Check sheet for the modelled part. Datum: model origin and axes. Units: mm. A direction names the side the tool comes from. Coordinates: 2 decimals unless noted, no trailing zeros. Loops run counter-clockwise (first coordinate to the right, second up) from the corner with the lowest first, then second, coordinate; pieces in that order, holes last.
```python
from build123d import *

# Parameters (mm, degrees)
SKETCH1_R              = 14.2875
SKETCH1_R_2            = 30
SKETCH1_R_3            = 15
SKETCH1_R_4            = 1.85
BOSS_EXTRUDE1_DEPTH    = 4
M3_5_CLEARANCE_HOLE1_D = 3.9
CUT_EXTRUDE1_DEPTH     = 10


with BuildPart() as part:
    # Sketch1 → Boss-Extrude1 (new body)
    with BuildSketch(Plane.XY):
        with BuildLine():
            Line((-228.151452703, 51.156245998), (232.657949662, 23.244899096))
            ThreePointArc((232.657949662, 23.244899096), (254.5375, 0), (232.657949662, -23.244899096))
            Line((232.657949662, -23.244899096), (-228.151452703, -51.156245998))
            ThreePointArc((-228.151452703, -51.156245998), (-282.5, 0), (-228.151452703, 51.156245998))
        make_face()
        with Locations((231.25, 0)):
            Circle(SKETCH1_R, mode=Mode.SUBTRACT)
        with Locations((-231.25, 0)):
            Circle(SKETCH1_R_2, mode=Mode.SUBTRACT)
        with Locations((-110.25, 0)):
            Circle(SKETCH1_R_3, mode=Mode.SUBTRACT)
        with Locations((-201.25, 44.517654426)):
            Circle(SKETCH1_R_4, mode=Mode.SUBTRACT)
        with Locations((-102.663346073, 38.546234825)):
            Circle(SKETCH1_R_4, mode=Mode.SUBTRACT)
        with Locations((-4.076692145, 32.574815224)):
            Circle(SKETCH1_R_4, mode=Mode.SUBTRACT)
        with Locations((94.509961782, 26.603395622)):
            Circle(SKETCH1_R_4, mode=Mode.SUBTRACT)
        with Locations((193.096615709, 20.631976021)):
            Circle(SKETCH1_R_4, mode=Mode.SUBTRACT)
        with Locations(Location((193.096615709, -20.631976021, 0), (0, 0, 180))):
            Circle(SKETCH1_R_4, mode=Mode.SUBTRACT)
        with Locations(Location((94.509961782, -26.603395622, 0), (0, 0, 180))):
            Circle(SKETCH1_R_4, mode=Mode.SUBTRACT)
        with Locations(Location((-4.076692145, -32.574815224, 0), (0, 0, 180))):
            Circle(SKETCH1_R_4, mode=Mode.SUBTRACT)
        with Locations(Location((-102.663346073, -38.546234825, 0), (0, 0, 180))):
            Circle(SKETCH1_R_4, mode=Mode.SUBTRACT)
        with Locations(Location((-201.25, -44.517654426, 0), (0, 0, 180))):
            Circle(SKETCH1_R_4, mode=Mode.SUBTRACT)
    extrude(amount=BOSS_EXTRUDE1_DEPTH)

    # M3.5 Clearance Hole1 (through all)
    with Locations(Plane.XY.offset(4)):
        with Locations((-231.25, 42.5), (-188.75, 0), (-132.75, 0), (-110.25, 22.5), (-87.75, 0), (-110.25, -22.5), (-273.75, 0), (-231.25, -42.5)):
            Hole(M3_5_CLEARANCE_HOLE1_D / 2)

    # Sketch7 → Cut-Extrude1 (cut)
    with BuildSketch(Plane.XY.offset(4)):
        with BuildLine():
            Line((108.094193191, 19.830412487), (152.959047941, 7.723728338))
            ThreePointArc((152.959047941, 7.723728338), (158.874816531, 0), (152.959047941, -7.723728338))
            Line((152.959047941, -7.723728338), (108.094193191, -19.830412487))
            ThreePointArc((108.094193191, -19.830412487), (101.145491167, -18.457819925), (98.009961782, -12.106684149))
            Line((98.009961782, -12.106684149), (98.009961782, 12.106684149))
            ThreePointArc((98.009961782, 12.106684149), (101.145491167, 18.457819925), (108.094193191, 19.830412487))
        make_face()
        with BuildLine():
            Line((91.009961782, -5.704410534), (91.009961782, 15.277961264))
            ThreePointArc((91.009961782, 15.277961264), (88.835311789, 20.761144399), (83.493637458, 23.263326493))
            Line((83.493637458, 23.263326493), (44.615483399, 25.618186527))
            ThreePointArc((44.615483399, 25.618186527), (36.490430728, 20.001229544), (40.014500476, 10.773682793))
            Line((40.014500476, 10.773682793), (78.892654535, -12.563549039))
            ThreePointArc((78.892654535, -12.563549039), (86.950871704, -12.666395092), (91.009961782, -5.704410534))
        make_face()
        with BuildLine():
            Line((11.040615102, 18.835101612), (59.256061992, -10.106989112))
            ThreePointArc((59.256061992, -10.106989112), (62.909345697, -18.868209702), (55.62243042, -24.951492846))
            Line((55.62243042, -24.951492846), (7.40698353, -27.871915166))
            ThreePointArc((7.40698353, -27.871915166), (1.440124719, -25.711899944), (-1.076692145, -19.886549937))
            Line((-1.076692145, -19.886549937), (-1.076692145, 11.975963107))
            ThreePointArc((-1.076692145, 11.975963107), (2.982397933, 18.937947665), (11.040615102, 18.835101612))
        make_face()
        with BuildLine():
            Line((-7.076692145, -16.488216766), (-7.076692145, 16.488216766))
            ThreePointArc((-7.076692145, 16.488216766), (-10.56107203, 23.091941092), (-17.978985888, 23.943194367))
            Line((-17.978985888, 23.943194367), (-60.331448304, 7.454977601))
            ThreePointArc((-60.331448304, 7.454977601), (-65.429154561, 0), (-60.331448304, -7.454977601))
            Line((-60.331448304, -7.454977601), (-17.978985888, -23.943194367))
            ThreePointArc((-17.978985888, -23.943194367), (-10.56107203, -23.091941092), (-7.076692145, -16.488216766))
        make_face()
        with BuildLine():
            Line((-79.023457852, 6.616651493), (-41.387349534, 21.268746715))
            ThreePointArc((-41.387349534, 21.268746715), (-38.261519247, 26.701886011), (-42.898985826, 30.918960984))
            Line((-42.898985826, 30.918960984), (-98.34861526, 34.277559647))
            ThreePointArc((-98.34861526, 34.277559647), (-103.531708107, 30.371987358), (-100.492037548, 24.638022826))
            ThreePointArc((-100.492037548, 24.638022826), (-91.408821848, 18.634913625), (-85.506059466, 9.486169241))
            ThreePointArc((-85.506059466, 9.486169241), (-82.861226958, 6.703913435), (-79.023457852, 6.616651493))
        make_face()
        with BuildLine():
            Line((-172.485050673, 29.401404781), (-141.465979865, 9.242335075))
            ThreePointArc((-141.465979865, 9.242335075), (-137.374294793, 8.625273291), (-134.218916995, 11.302257212))
            ThreePointArc((-134.218916995, 11.302257212), (-127.488882583, 20.126373923), (-117.7355471, 25.420790401))
            ThreePointArc((-117.7355471, 25.420790401), (-114.065979457, 30.952175342), (-118.881140508, 35.52122011))
            Line((-118.881140508, 35.52122011), (-169.458127675, 38.584681548))
            ThreePointArc((-169.458127675, 38.584681548), (-174.509115504, 35.159056133), (-172.485050673, 29.401404781))
        make_face()
        with BuildLine():
            Line((-192.622687213, 24.889664687), (-187.500750367, 6.648335526))
            ThreePointArc((-187.500750367, 6.648335526), (-185.706988459, 4.01513348), (-182.686915809, 3))
            Line((-182.686915809, 3), (-159.740638738, 3))
            ThreePointArc((-159.740638738, 3), (-154.946782383, 6.579105474), (-157.016013037, 12.192423498))
            Line((-157.016013037, 12.192423498), (-185.084226954, 30.43375266))
            ThreePointArc((-185.084226954, 30.43375266), (-190.771187254, 30.269303059), (-192.622687213, 24.889664687))
        make_face()
        with BuildLine():
            Line((-118.881140508, -35.52122011), (-169.458127675, -38.584681548))
            ThreePointArc((-169.458127675, -38.584681548), (-174.509115504, -35.159056133), (-172.485050673, -29.401404781))
            Line((-172.485050673, -29.401404781), (-141.465979865, -9.242335075))
            ThreePointArc((-141.465979865, -9.242335075), (-137.374294793, -8.625273291), (-134.218916995, -11.302257212))
            ThreePointArc((-134.218916995, -11.302257212), (-127.488882583, -20.126373923), (-117.7355471, -25.420790401))
            ThreePointArc((-117.7355471, -25.420790401), (-114.065979457, -30.952175342), (-118.881140508, -35.52122011))
        make_face()
        with BuildLine():
            Line((-157.016013037, -12.192423498), (-185.084226954, -30.43375266))
            ThreePointArc((-185.084226954, -30.43375266), (-190.771187254, -30.269303059), (-192.622687213, -24.889664687))
            Line((-192.622687213, -24.889664687), (-187.500750367, -6.648335526))
            ThreePointArc((-187.500750367, -6.648335526), (-185.706988459, -4.01513348), (-182.686915809, -3))
            Line((-182.686915809, -3), (-159.740638738, -3))
            ThreePointArc((-159.740638738, -3), (-154.946782383, -6.579105474), (-157.016013037, -12.192423498))
        make_face()
        with BuildLine():
            Line((-42.898985826, -30.918960984), (-98.34861526, -34.277559647))
            ThreePointArc((-98.34861526, -34.277559647), (-103.531708107, -30.371987358), (-100.492037548, -24.638022826))
            ThreePointArc((-100.492037548, -24.638022826), (-91.408821848, -18.634913625), (-85.506059466, -9.486169241))
            ThreePointArc((-85.506059466, -9.486169241), (-82.861226958, -6.703913435), (-79.023457852, -6.616651493))
            Line((-79.023457852, -6.616651493), (-41.387349534, -21.268746715))
            ThreePointArc((-41.387349534, -21.268746715), (-38.261519247, -26.701886011), (-42.898985826, -30.918960984))
        make_face()
    extrude(amount=-CUT_EXTRUDE1_DEPTH, mode=Mode.SUBTRACT)


solid = part.part
```
1) Section check B-B on x = 27.5. Enter the section's corners in (y, z).
Answer sheet:
outline: (-35.67, 0) - (-26.65, 0) - (-26.65, 4) - (-35.67, 4) - close; (8.96, 0) - (35.67, 0) - (35.67, 4) - (8.96, 4) - close
2) Depth check by flat-ended pin: pin 1 (6 mm diameter, centred on x = -188.75, y = 0, fed in from -Z); pin 2 (3.5 mm diameter, centred on x = 94.51, y = -26.6, fed in from -Z); pin 3 (1.2 mm diameter, centred on x = -175, z = 2.5, fed in from +Y). Enter the tip coordinate at first touch or a pass-through.
Answer sheet:
pin 1: stops at z = 0
pin 2: passes through
pin 3: stops at y = 47.97
3) Mould release check, pull along Y, two halves, no side actions. Record for faces 3 (the cylindrical face through (-202.635, 9.011, 1.972)), 4 (the flat face through (-70, 1, 0)), 5 (the flat face through (-0.972, 37.396, 1.972)): +Y half, -Y half, draft (parallel to the pull), parting line (faces both ways), or undercut.
Answer sheet:
face 3: undercut
face 4: draft
face 5: +Y half
4) Section check A-A on x = -49.5. Enter the section's corners in (y, z), plus the area to 3 significant figures.
Answer sheet:
outline: (-40.34, 0) - (-31.32, 0) - (-31.32, 4) - (-40.34, 4) - close; (-18.11, 0) - (-11.67, 0) - (-11.67, 4) - (-18.11, 4) - close; (11.67, 0) - (18.11, 0) - (18.11, 4) - (11.67, 4) - close; (31.32, 0) - (40.34, 0) - (40.34, 4) - (31.32, 4) - close
area: 124 mm2
5) Section check D-D on x = 186.5. Enter the section's corners in (y, z), plus the area to 3 significant figures.
Answer sheet:
outline: (-26.04, 0) - (26.04, 0) - (26.04, 4) - (-26.04, 4) - close
area: 208 mm2
6) Scan lines: line 1 (Y direction, x = -231.25, z = 1.7); line 2 (Y direction, x = -39, z = 0.4); line 3 (Y direction, x = -168, z = 1.65). Record each from-to range of solid material in increasing order.
Answer sheet:
line 1: y = -51.25 to -44.45, -40.55 to -30, 30 to 40.55, 44.45 to 51.25
line 2: y = -39.7 to -28.64, -23.22 to -15.76, 15.76 to 23.22, 28.64 to 39.7
line 3: y = -47.51 to -38.5, -26.49 to -19.33, -3 to 3, 19.33 to 26.49, 38.5 to 47.51
7) Set-up check for faces 1 (the flat face through (-70, 1, 4)), 2 (the flat face through (-170.854, -21.185, 2.028)): record each of +Z, -Z, +X, -X, +Y, -Y from which the full face is reachable in a straight line by a thin tool's end or side.
Answer sheet:
face 1: +Z, +X, -X, +Y, -Y
face 2: +Z, -Z
8) Section check C-C on z = 3.25. Give the number of separate pieces and of enclosed holes in the cut face, plus the area to 3 significant figures.
Answer sheet:
separate pieces: 1
enclosed holes: 31
area: 22,400 mm2
